Read the model definition and answer for the solid it produces. Units are mm, in the model's axes. Face numbers are marked on the shaded views. Coordinates: 2 decimals unless noted, no trailing zeros. Write each loop counter-clockwise with the first axis right and the second up, starting at its lowest first coordinate (ties: lowest second). Pieces come first, ordered by that corner, then holes. Notation, with made-up numbers: (21, 53.5) -> (30, 53.5) arc R17 ccw to (30, 63.5) -> close; hole circle Ø5 at (-28.5, -29.75). An arc over 180 degrees is marked (long way). Write item = value, one per line. Start each with the question number.
1) For a pull along X with two mould halves and no side action, classify the marked faces 1, 2 and 3 as released by +X, released by -X, zero draft, split by the parting line, or undercut.
2) Section B-B (y = 11) is taken. Determine the outline of the cut face in (x, z), plus the area to 3 significant figures.
3) Section D-D (y = 1) is taken. Determine the outline of the cut face in (x, z).
4) Section A-A (x = 0) is taken. Determine the outline of the cut face in (y, z).
5) Flat-ended cylindrical pins translate along their axes: pin 1 Ø3 at (x, y) = (-2.5, 10) entering from -Z; pin 2 Ø2 at (x, y) = (0.5, 8) entering from -Z; pin 3 Ø2 at (x, z) = (0, 8.5) entering from -Y. Find the tip coordinate at first contact, or state that the pin passes through.
6) Find the intervals of material crossed by line 1 along Z through (x, y) = (0, 7.25); line 2 along Y through (x, z) = (6.25, -3.5); line 3 along Z through (x, y) = (-1, 5), in increasing order. Write a range as from..to.
7) Section C-C (z = 21.5) is taken. Determine the outline of the cut face in (x, y).
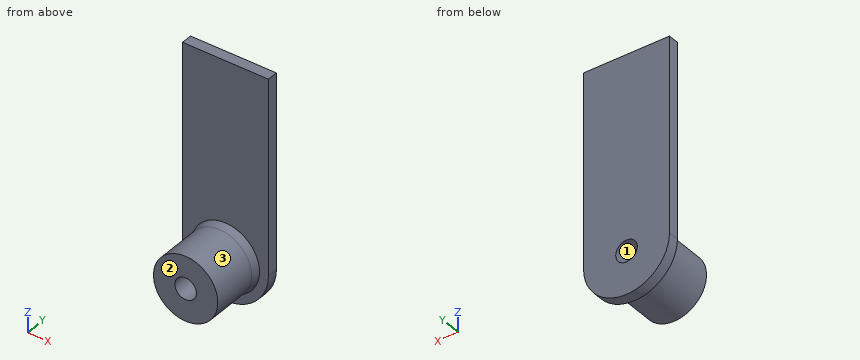
from build123d import *

# Parameters (mm, degrees)
SKETCH1_R           = 5.95
BOSS_EXTRUDE1_DEPTH = 10
BOSS_EXTRUDE2_DEPTH = 2
CHAMFER1_SIZE       = 1.5
CHAMFER1_SIZE2      = 0.346302287
SKETCH3_R           = 2
CUT_EXTRUDE1_DEPTH  = 13
SKETCH4_W           = 15.9
SKETCH4_H           = 2
BOSS_EXTRUDE3_DEPTH = 20


with BuildPart() as part:
    # Sketch1 → Boss-Extrude1 (new body)
    with BuildSketch(Plane(origin=(0, 0, 0), x_dir=(1, 0, 0), z_dir=(0, 1, 0))):
        Circle(SKETCH1_R)
    extrude(amount=BOSS_EXTRUDE1_DEPTH)

    # Sketch2 → Boss-Extrude2 (add)
    with BuildSketch(Plane(origin=(0, 10, 0), x_dir=(1, 0, 0), z_dir=(0, 1, 0))):
        with BuildLine():
            Line((-7.95, 0), (-7.95, -16))
            Line((-7.95, -16), (7.95, -16))
            Line((7.95, -16), (7.95, 0))
            ThreePointArc((7.95, 0), (0, 7.95), (-7.95, 0))
        make_face()
    extrude(amount=BOSS_EXTRUDE2_DEPTH)

    # Chamfer1
    chamfer1_edges = [part.edges().sort_by_distance(p)[0] for p in [
        (-5.95, 10, 0),
    ]]
    chamfer1_side = [part.faces().sort_by_distance(p)[0] for p in [
        (-5.95, 5, 0),
    ]]
    chamfer(chamfer1_edges, length=CHAMFER1_SIZE, length2=CHAMFER1_SIZE2, reference=chamfer1_side[0])

    # Sketch3 → Cut-Extrude1 (cut, through all)
    with BuildSketch(Plane.XZ):
        Circle(SKETCH3_R)
    extrude(amount=-CUT_EXTRUDE1_DEPTH, mode=Mode.SUBTRACT)

    # Sketch4 → Boss-Extrude3 (add)
    with BuildSketch(Plane.XY.offset(16)):
        with Locations((0, 11)):
            Rectangle(SKETCH4_W, SKETCH4_H)
    extrude(amount=BOSS_EXTRUDE3_DEPTH)


solid = part.part
Answer key:
q1.face_1 = undercut
q1.face_2 = zero draft
q1.face_3 = split by the parting line
q2.outline = (-7.95, 0) arc R7.95 ccw to (7.95, 0) -> (7.95, 36) -> (-7.95, 36) -> close; hole circle Ø4 at (0, 0)
q2.area = 659 mm^2
q3.outline = circle Ø11.9 at (0, 0); hole circle Ø4 at (0, 0)
q4.outline = (0, -5.95) -> (8.5, -5.95) -> (10, -6.3) -> (10, -7.95) -> (12, -7.95) -> (12, -2) -> (0, -2) -> close; (0, 2) -> (12, 2) -> (12, 36) -> (10, 36) -> (10, 6.3) -> (8.5, 5.95) -> (0, 5.95) -> close
q5.pin_1 = -7.89
q5.pin_2 = -6.05
q5.pin_3 = 10
q6.line_1 = -5.95..-2, 2..5.95
q6.line_2 = 10..12
q6.line_3 = -5.87..-1.73, 1.73..5.87
q7.outline = (-7.95, 10) -> (7.95, 10) -> (7.95, 12) -> (-7.95, 12) -> close
